Part model, mm, in its own coordinate system. Face numbers are marked on the shaded views. Give positions to 0.01 mm unless a question says otherwise; leave off trailing zeros. Write each loop counter-clockwise with the first axis right and the second up, starting at its lowest first coordinate (ties: lowest second). Pieces come first, ordered by that corner, then holes.
```python
from build123d import *

# Parameters (mm, degrees)
SKETCH1_W           = 14
SKETCH1_H           = 14
SKETCH1_W_2         = 10
SKETCH1_H_2         = 10
BOSS_EXTRUDE1_DEPTH = 12
SKETCH2_R           = 9.5
CUT_EXTRUDE1_DEPTH  = 30
BOSS_EXTRUDE2_DEPTH = 30
BOSS_EXTRUDE3_DEPTH = 32.5
CUT_EXTRUDE2_DEPTH  = 79.125958548
CUT_EXTRUDE3_DEPTH  = 32.5
BOSS_EXTRUDE4_DEPTH = 32.5


with BuildPart() as part:
    # Sketch1 → Boss-Extrude1 (new body)
    with BuildSketch(Plane.XY):
        Rectangle(SKETCH1_W, SKETCH1_H)
        Rectangle(SKETCH1_W_2, SKETCH1_H_2, mode=Mode.SUBTRACT)
    extrude(amount=BOSS_EXTRUDE1_DEPTH)

    # Sketch2 → Cut-Extrude1 (cut)
    with BuildSketch(Plane(origin=(7, 0, 0), x_dir=(0, 0, -1), z_dir=(1, 0, 0))):
        Circle(SKETCH2_R)
    extrude(amount=-CUT_EXTRUDE1_DEPTH, mode=Mode.SUBTRACT)

    # Sketch4 → Boss-Extrude2 (add, symmetric)
    with BuildSketch(Plane(origin=(0, 0, 0), x_dir=(1, 0, 0), z_dir=(0, 1, 0))):
        Polygon((-7, -12), (-29.981333294, -31.283628291), (-32.293968462, -31.283628291), (-7, -10.059468683), align=None)
        Polygon((7, -10.059468683), (7, -12), (29.981333294, -31.283628291), (32.293968462, -31.283628291), align=None)
    extrude(amount=BOSS_EXTRUDE2_DEPTH, both=True)

    # Sketch6 → Boss-Extrude3 (add, symmetric)
    with BuildSketch(Plane(origin=(0, 0, 0), x_dir=(0, 0, -1), z_dir=(1, 0, 0))):
        Polygon((-10.059468683, -7), (-12, -7), (-31.283628291, -30), (-29.343096974, -30), align=None)
        Polygon((-31.283628291, 30), (-29.343096974, 30), (-10.059468683, 7), (-12, 7), align=None)
    extrude(amount=BOSS_EXTRUDE3_DEPTH, both=True)

    # Sketch7 → Cut-Extrude2 (cut, through all)
    with BuildSketch(Plane(origin=(32.5, 0, 0), x_dir=(0, 0, -1), z_dir=(1, 0, 0))):
        Polygon((-29.343096974, 30), (-10.059468683, 7), (-10.059468683, 30), align=None)
        Polygon((-29.343096974, -30), (-10.059468683, -7), (-10.059468683, -30), align=None)
    extrude(amount=-CUT_EXTRUDE2_DEPTH, mode=Mode.SUBTRACT)

    # Sketch9 → Cut-Extrude3 (cut, symmetric)
    with BuildSketch(Plane(origin=(0, 0, 0), x_dir=(1, 0, 0), z_dir=(0, 1, 0))):
        Polygon((-32.5, -31.283628291), (-7, -10.059468683), (-32.5, -10.059468683), align=None)
        Polygon((7, -10.059468683), (32.5, -10.059468683), (32.5, -31.283628291), align=None)
    extrude(amount=CUT_EXTRUDE3_DEPTH, both=True, mode=Mode.SUBTRACT)

    # Sketch10 → Boss-Extrude4 (add, symmetric)
    with BuildSketch(Plane(origin=(0, 0, 0), x_dir=(0, 0, -1), z_dir=(1, 0, 0))):
        Polygon((-31.283628291, -30), (-29.343096974, -30), (-31.283628291, -32.314513618), align=None)
        Polygon((-29.343096974, 30), (-31.283628291, 32.314513618), (-31.283628291, 30), align=None)
    extrude(amount=BOSS_EXTRUDE4_DEPTH, both=True)


solid = part.part
```
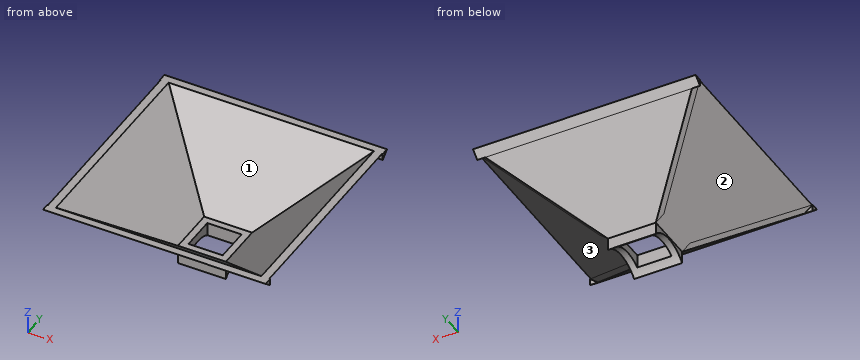
1) Saw through at D-D, the plane y = -13. Write the cut outline in (x, z).
Answers follow:
outline: (-32.29, 31.28) - (-15.31, 17.03) - (-15.38, 17.03) - (-13.04, 15.09) - (13.04, 15.09) - (15.38, 17.03) - (15.31, 17.03) - (32.29, 31.28) - (29.98, 31.28) - (13, 17.03) - (-13, 17.03) - (-29.98, 31.28) - close
2) Saw through at A-A, the plane x = 3. Write the cut outline in (y, z), then the cut area to 3 significant figures.
Answers follow:
outline: (-32.31, 31.28) - (-7, 10.06) - (-7, 6.42) arc R9.5 cw to (-5, 8.08) - (-5, 12) - (-7, 12) - (-30, 31.28) - close; (5, 8.08) arc R9.5 cw to (7, 6.42) - (7, 10.06) - (32.31, 31.28) - (30, 31.28) - (7, 12) - (5, 12) - close
area: 112 mm2
3) Pin check, flat tips, straight feed: pin 1 Ø3 at (y, z) = (0, 9) entering from -X (3 decimals); pin 2 Ø2 at (x, z) = (1, 11) entering from +Y; pin 3 Ø2 at (x, z) = (8, 11) entering from -Y; pin 4 Ø1.1 at (y, z) = (1, 7.5) entering from +X. Stop position of each tip, or through.
Answers follow:
pin 1: stops at x = -7.525
pin 2: stops at y = 9.31
pin 3: stops at y = -9.31
pin 4: passes through
4) Wall check: L1, parallel to Y at x = 12, z = 26.75; L2, parallel to Y at x = 20.5, z = 29; L3, parallel to X at y = -5.5, z = 27.75. Give the ranges that are in metal, low to high.
Answers follow:
L1: y = -26.91 to -24.59, 24.59 to 26.91
L2: y = -29.59 to -27.28, 27.28 to 29.59
L3: x = -28.08 to -25.77, 25.77 to 28.08
5) Saw through at C-C, the plane x = -6. Write the cut outline in (y, z), then the cut area to 3 significant figures.
Answers follow:
outline: (-32.31, 31.28) - (-7, 10.06) - (-7, 6.42) arc R9.5 cw to (7, 6.42) - (7, 10.06) - (32.31, 31.28) - (30, 31.28) - (7, 12) - (-7, 12) - (-30, 31.28) - close
area: 142 mm2
6) Two-plate mould, pull along X, no slides. Class the marked faces 1, 2 and 3: +X half, -X half, draft (parallel to the pull), parting line (faces both ways), or undercut.
Answers follow:
face 1: undercut
face 2: -X half
face 3: +X half
